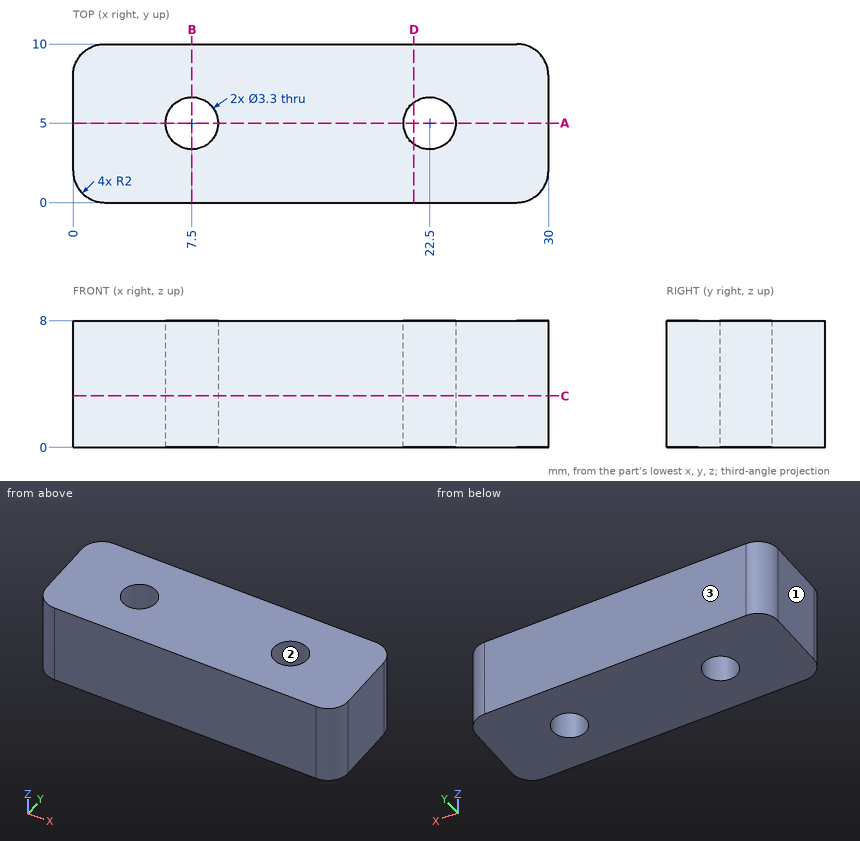
Here's the drawing with two shaded views (mm, measured from the low corner). I have some questions. Give positions to 0.01 mm unless a question says otherwise; leave off trailing zeros. Order: outer loops, then holes, each group sorted by start corner. A loop starts at its lowest first (then second) coordinate and runs counter-clockwise, first axis right, second up.
Q1. We'd pull the mould along Y, two halves only. Please class the marked faces 1, 2 and 3: +Y half, -Y half, draft (parallel to the pull), parting line (faces both ways), or undercut.
Q2. Suppose I cut it at A-A, the plane y = 5. Write out the boundary of the cut face in (x, z), and give its area (3 significant figures).
Q3. Suppose I cut it at D-D, the plane x = 21.5. Write out the boundary of the cut face in (y, z), and give its area (3 significant figures).
Q4. If I drill on line 1 along Y through (x, z) = (7.5, 6.5); line 2 along X through (y, z) = (5.25, 3.5); line 3 along X through (y, z) = (4.25, 7.75), over which ranges is the centre line in solid material (lowest first)?
Q5. Suppose I cut it at B-B, the plane x = 7.5. Write out the boundary of the cut face in (y, z).
Q6. Suppose I cut it at C-C, the plane z = 3.25. Write out the boundary of the cut face in (x, y), and give its area (3 significant figures).
Solution:
1. face 1: draft
1. face 2: undercut
1. face 3: +Y half
2. outline: (0, 0) - (5.85, 0) - (5.85, 8) - (0, 8) - close; (9.15, 0) - (20.85, 0) - (20.85, 8) - (9.15, 8) - close; (24.15, 0) - (30, 0) - (30, 8) - (24.15, 8) - close
2. area: 187 mm2
3. outline: (0, 0) - (3.69, 0) - (3.69, 8) - (0, 8) - close; (6.31, 0) - (10, 0) - (10, 8) - (6.31, 8) - close
3. area: 59.0 mm2
4. line 1: y = 0 to 3.35, 6.65 to 10
4. line 2: x = 0 to 5.87, 9.13 to 20.87, 24.13 to 30
4. line 3: x = 0 to 6.03, 8.97 to 21.03, 23.97 to 30
5. outline: (0, 0) - (3.35, 0) - (3.35, 8) - (0, 8) - close; (6.65, 0) - (10, 0) - (10, 8) - (6.65, 8) - close
6. outline: (0, 2) arc R2 ccw to (2, 0) - (28, 0) arc R2 ccw to (30, 2) - (30, 8) arc R2 ccw to (28, 10) - (2, 10) arc R2 ccw to (0, 8) - close; hole circle Ø3.3 at (7.5, 5); hole circle Ø3.3 at (22.5, 5)
6. area: 279 mm2
